from build123d import *

# Parameters (mm, degrees)
IZIM1_W                     = 130
IZIM1_H                     = 120
Y_KSEKLIK_EKSTR_ZYON1_DEPTH = 5
IZIM1_3_W                   = 140
IZIM1_3_H                   = 130
IZIM1_3_W_2                 = 130
IZIM1_3_H_2                 = 120
Y_KSEKLIK_EKSTR_ZYON2_DEPTH = 55
RADYUS1_R                   = 8
RADYUS2_R                   = 2


with BuildPart() as part:
    # Çizim1 → Yükseklik-Ekstrüzyon1 (new body)
    with BuildSketch(Plane(origin=(0, 0, 0), x_dir=(0, 1, 0), z_dir=(0, 0, 1))):
        with Locations((70, 65)):
            Rectangle(IZIM1_W, IZIM1_H)
    extrude(amount=Y_KSEKLIK_EKSTR_ZYON1_DEPTH)

    # Çizim1<3> → Yükseklik-Ekstrüzyon2 (add)
    with BuildSketch(Plane(origin=(0, 0, 0), x_dir=(0, 1, 0), z_dir=(0, 0, 1))):
        with Locations((70, 65)):
            Rectangle(IZIM1_3_W, IZIM1_3_H)
        with Locations((70, 65)):
            Rectangle(IZIM1_3_W_2, IZIM1_3_H_2, mode=Mode.SUBTRACT)
    extrude(amount=Y_KSEKLIK_EKSTR_ZYON2_DEPTH)

    # Radyus1
    radyus1_edges = [part.edges().sort_by_distance(p)[0] for p in [
        (-125, 70, 5),
        (-5, 135, 30),
        (-125, 135, 30),
        (-125, 5, 30),
        (-5, 5, 30),
        (-65, 5, 5),
        (-5, 70, 5),
        (-65, 135, 5),
    ]]
    fillet(radyus1_edges, radius=RADYUS1_R)

    # Radyus2
    radyus2_edges = [part.edges().sort_by_distance(p)[0] for p in [
        (-5, 70, 55),
        (-65, 135, 55),
        (-125, 70, 55),
        (-65, 5, 55),
        (-7.343145751, 132.656854249, 55),
        (-122.656854249, 132.656854249, 55),
        (-122.656854249, 7.343145751, 55),
        (-7.343145751, 7.343145751, 55),
    ]]
    fillet(radyus2_edges, radius=RADYUS2_R)


solid = part.part
Geometry check sheet. Reference: the model listing, model coordinates, mm. A direction names the side the tool comes from. Coordinates: 2 decimals unless noted, no trailing zeros. Order: outer loops, then holes, each group sorted by start corner. A loop starts at its lowest first (then second) coordinate and runs counter-clockwise, first axis right, second up. Notation, with made-up numbers: (21, 30) - (80, 30) arc R16 ccw to (80, 37) - close; hole circle Ø4 at (54, -12.5). An arc over 180 degrees is marked (long way). Answer in a Markdown table with one row per item. Add a question column.
1) Cross-section at A-A, the plane z = 27. Record the cut outline in (x, y).
2) Material ranges on line 1 along Y through (x, z) = (-89.5, 42); line 2 along X through (y, z) = (56.5, 51); line 3 along Z through (x, y) = (-66.5, 17), recorded low to high. Write a range as [from, to].
3) Cross-section at C-C, the plane x = -109.5. Record the cut outline in (y, z), then the cut area to 3 significant figures.
4) Cross-section at B-B, the plane y = 123.5. Record the cut outline in (x, z).
5) Release check for a two-part mould opening along X. For faces 3 (the flat face through (-2.7, 64.5, 55)), 4 (the flat face through (0, 69, 27)), 5 (the flat face through (-130, 69, 27)), 6 (the cylindrical face through (-65.728, 7.281, 7.406)) record: +X half, -X half, draft (parallel to the pull), parting line (faces both ways), or undercut.
6) Set-up check for faces 1 (the flat face through (-64, 140, 27)), 2 (the flat face through (-66, 69, 5)): record each of +Z, -Z, +X, -X, +Y, -Y from which the full face is reachable in a straight line by a thin tool's end or side.
7) Gauge pin test, flat end, axial feed: P1, Ø5, axis at x = -117, y = 89, coming from the +Z side. Record the tip position at first contact, or that the pin passes through.
Check result:
| question | item | result |
|---|---|---|
| 1 | outline | (-130, 0) - (0, 0) - (0, 140) - (-130, 140) - close; hole (-125, 13) arc R8 ccw to (-117, 5) - (-13, 5) arc R8 ccw to (-5, 13) - (-5, 127) arc R8 ccw to (-13, 135) - (-117, 135) arc R8 ccw to (-125, 127) - close |
| 2 | line 1 | y = [0, 5], [135, 140] |
| 2 | line 2 | x = [-130, -125], [-5, 0] |
| 2 | line 3 | z = [0, 5] |
| 3 | outline | (0, 0) - (140, 0) - (140, 55) - (137, 55) arc R2 ccw to (135, 53) - (135, 13) arc R8 cw to (127, 5) - (13, 5) arc R8 cw to (5, 13) - (5, 53) arc R2 ccw to (3, 55) - (0, 55) - close |
| 3 | area | 1,230 mm² |
| 4 | outline | (-130, 0) - (0, 0) - (0, 55) - (-3, 55) arc R2 ccw to (-5, 53) - (-5, 13) arc R8 cw to (-13, 5) - (-117, 5) arc R8 cw to (-125, 13) - (-125, 53) arc R2 ccw to (-127, 55) - (-130, 55) - close |
| 5 | face 3 | draft |
| 5 | face 4 | +X half |
| 5 | face 5 | -X half |
| 5 | face 6 | undercut |
| 6 | face 1 | +Z, -Z, +X, -X, +Y |
| 6 | face 2 | +Z |
| 7 | P1 | stops at z = 5.4 |
